Input: part model. Units: mm. Frame: model coordinates. A direction names the side the tool comes from. Round coordinates to 2 decimals unless told otherwise and drop trailing zeros. Write each loop counter-clockwise with the first axis right and the second up, starting at its lowest first coordinate (ties: lowest second). Pieces come first, ordered by that corner, then holes. Notation, with made-up numbers: (72, 28) - (131, 28) arc R17 cw to (131, 60) - close; hole circle Ø9 at (-19, 87.25). An arc over 180 degrees is marked (long way). One line per item, written item: value. Start each with the question number.
```python
from build123d import *

# Parameters (mm, degrees)
SKETCH_1_W      = 82.6
SKETCH_1_H      = 62
EXTRUDE_1_DEPTH = 25
SKETCH_2_W      = 68
SKETCH_2_H      = 12
EXTRUDE_2_DEPTH = 1
FILLET_1_R      = 1
SKETCH_3_R      = 3
EXTRUDE_3_DEPTH = 5.5
SKETCH_4_W      = 10
SKETCH_4_H      = 15
EXTRUDE_4_DEPTH = 11
SKETCH_5_W      = 31
SKETCH_5_H      = 12.5
EXTRUDE_5_DEPTH = 5
EXTRUDE_6_DEPTH = 15
FILLET_2_R      = 1
SKETCH_7_W      = 7
SKETCH_7_H      = 7
EXTRUDE_7_DEPTH = 12.5


with BuildPart() as part:
    # 草图1 → 凸台-拉伸1 (new body)
    with BuildSketch(Plane(origin=(0, 0, 0), x_dir=(1, 0, 0), z_dir=(0, 1, 0))):
        Rectangle(SKETCH_1_W, SKETCH_1_H)
    extrude(amount=EXTRUDE_1_DEPTH)

    # 草图2 → 凸台-拉伸2 (add)
    # profile 1 of 2: a face of its own
    with BuildSketch(Plane.XZ):
        with Locations((0, 37)):
            Rectangle(SKETCH_2_W, SKETCH_2_H)
        with BuildLine():
            Line((-29, 39.5), (-21, 39.5))
            ThreePointArc((-21, 39.5), (-19, 37.5), (-21, 35.5))
            Line((-21, 35.5), (-29, 35.5))
            ThreePointArc((-29, 35.5), (-31, 37.5), (-29, 39.5))
        make_face(mode=Mode.SUBTRACT)
        with BuildLine():
            Line((21, 39.5), (29, 39.5))
            ThreePointArc((29, 39.5), (31, 37.5), (29, 35.5))
            Line((29, 35.5), (21, 35.5))
            ThreePointArc((21, 35.5), (19, 37.5), (21, 39.5))
        make_face(mode=Mode.SUBTRACT)
        with BuildLine():
            Line((-5.5, 39.5), (-2, 39.5))
            ThreePointArc((-2, 39.5), (0, 41.5), (2, 39.5))
            Line((2, 39.5), (5.5, 39.5))
            ThreePointArc((5.5, 39.5), (7.5, 37.5), (5.5, 35.5))
            Line((5.5, 35.5), (2, 35.5))
            ThreePointArc((2, 35.5), (0, 33.5), (-2, 35.5))
            Line((-2, 35.5), (-5.5, 35.5))
            ThreePointArc((-5.5, 35.5), (-7.5, 37.5), (-5.5, 39.5))
        make_face(mode=Mode.SUBTRACT)
    # profile 2 of 2: a face of its own
    with BuildSketch(Plane.XZ):
        with Locations((0, -37)):
            Rectangle(SKETCH_2_W, SKETCH_2_H)
        with BuildLine():
            Line((2, -35.5), (5.5, -35.5))
            ThreePointArc((5.5, -35.5), (7.5, -37.5), (5.5, -39.5))
            Line((5.5, -39.5), (2, -39.5))
            ThreePointArc((2, -39.5), (0, -41.5), (-2, -39.5))
            Line((-2, -39.5), (-5.5, -39.5))
            ThreePointArc((-5.5, -39.5), (-7.5, -37.5), (-5.5, -35.5))
            Line((-5.5, -35.5), (-2, -35.5))
            ThreePointArc((-2, -35.5), (0, -33.5), (2, -35.5))
        make_face(mode=Mode.SUBTRACT)
        with BuildLine():
            Line((21, -39.5), (29, -39.5))
            ThreePointArc((29, -39.5), (31, -37.5), (29, -35.5))
            Line((29, -35.5), (21, -35.5))
            ThreePointArc((21, -35.5), (19, -37.5), (21, -39.5))
        make_face(mode=Mode.SUBTRACT)
        with BuildLine():
            Line((-29, -39.5), (-21, -39.5))
            ThreePointArc((-21, -39.5), (-19, -37.5), (-21, -35.5))
            Line((-21, -35.5), (-29, -35.5))
            ThreePointArc((-29, -35.5), (-31, -37.5), (-29, -39.5))
        make_face(mode=Mode.SUBTRACT)
    extrude(amount=-EXTRUDE_2_DEPTH)

    # 圆角1
    fillet_1_edges = [part.edges().sort_by_distance(p)[0] for p in [
        (0, 1, 31),
        (0, 1, -31),
    ]]
    fillet(fillet_1_edges, radius=FILLET_1_R)

    # 草图3 → 凸台-拉伸3 (add)
    with BuildSketch(Plane(origin=(41.3, 0, 0), x_dir=(0, 0, -1), z_dir=(1, 0, 0))):
        with Locations(Location((-12.5, 12, 0), (0, 0, 180))):
            Circle(SKETCH_3_R)
    extrude(amount=EXTRUDE_3_DEPTH)

    # 草图4 → 凸台-拉伸4 (add)
    with BuildSketch(Plane(origin=(41.3, 0, 0), x_dir=(0, 0, -1), z_dir=(1, 0, 0))):
        with Locations((3, 14)):
            Rectangle(SKETCH_4_W, SKETCH_4_H)
    extrude(amount=EXTRUDE_4_DEPTH)

    # 草图5 → 凸台-拉伸5 (add)
    with BuildSketch(Plane.ZY.offset(41.3)):
        with Locations((8.5, 13.05)):
            Rectangle(SKETCH_5_W, SKETCH_5_H)
    extrude(amount=EXTRUDE_5_DEPTH)

    # 草图6 → 凸台-拉伸6 (add)
    with BuildSketch(Plane.ZY.offset(46.3)):
        Polygon((-1, 18.3), (18, 18.3), (16.5, 7.8), (0.5, 7.8), align=None)
    extrude(amount=EXTRUDE_6_DEPTH)

    # 圆角2
    fillet_2_edges = [part.edges().sort_by_distance(p)[0] for p in [
        (-53.8, 18.3, -1),
        (-53.8, 7.8, 0.5),
        (-53.8, 7.8, 16.5),
        (-53.8, 18.3, 18),
    ]]
    fillet(fillet_2_edges, radius=FILLET_2_R)

    # 草图7 → 凸台-拉伸7 (add)
    with BuildSketch(Plane(origin=(46.8, 0, 0), x_dir=(0, 0, -1), z_dir=(1, 0, 0))):
        with Locations((-12.5, 12)):
            Rectangle(SKETCH_7_W, SKETCH_7_H)
    extrude(amount=EXTRUDE_7_DEPTH)


solid = part.part
```
Q1. Access query for faces 1 (the flat face through (-54, 7.8, 9)), 2 (the cylindrical face through (44, 11.9, 9.5)), 3 (the flat face through (52.3, 14, -3)), 4 (the flat face through (-44, 13, 24)), 5 (the flat face through (-44, 19.3, 8)). Directions: +Z, -Z, +X, -X, +Y, -Y. A direction counts if a zero-diameter tool reaches every point of the face in a straight line with its end or side. Return the directions, or none.
Q2. Cut plane D-D, the plane z = -19. Output: boundary loops of the cut face in (x, y).
Q3. Cut plane B-B, the plane z = -37.5. Output: boundary loops of the cut face in (x, y).
Q4. Contact query for flat-ended pins moving along their axis: pin 1 Ø1 at (x, y) = (24.5, 12) entering from +Z; pin 2 Ø6 at (x, y) = (-2.5, 4.5) entering from +Z; pin 3 Ø7.5 at (x, y) = (54, 11) entering from -Z. Output: stop coordinate, or through.
Q5. Cut plane C-C, the plane y = 12. Output: boundary loops of the cut face in (x, z).
Q6. Material intervals for probe 1 along X at (y, z) = (16.5, 27); probe 2 along Z at (x, y) = (37, 16.25); probe 3 along Y at (x, z) = (-45, 4), sorted ascending. Write a range as from..to.
Q7. Cut plane A-A, the plane x = -26. Output: boundary loops of the cut face in (y, z), and give its area (3 significant figures).
A:
1. face 1: +Z, -Z, -X, -Y
1. face 2: none
1. face 3: -Z, +X, +Y, -Y
1. face 4: +Z, -X, +Y, -Y
1. face 5: +Z, -Z, -X, +Y
2. outline: (-41.3, 0) - (41.3, 0) - (41.3, 25) - (-41.3, 25) - close
3. outline: (-34, 0) - (-31, 0) - (-31, 1) - (-34, 1) - close; (-19, 0) - (-7.5, 0) - (-7.5, 1) - (-19, 1) - close; (7.5, 0) - (19, 0) - (19, 1) - (7.5, 1) - close; (31, 0) - (34, 0) - (34, 1) - (31, 1) - close
4. pin 1: stops at z = 31
4. pin 2: stops at z = 31.13
4. pin 3: stops at z = -8
5. outline: (-61.3, -0.1) - (-46.3, -0.1) - (-46.3, -7) - (-41.3, -7) - (-41.3, -31) - (41.3, -31) - (41.3, -8) - (52.3, -8) - (52.3, 2) - (41.3, 2) - (41.3, 9.5) - (46.8, 9.5) - (46.8, 9) - (59.3, 9) - (59.3, 16) - (46.8, 16) - (46.8, 15.5) - (41.3, 15.5) - (41.3, 31) - (-41.3, 31) - (-41.3, 24) - (-46.3, 24) - (-46.3, 17.1) - (-61.3, 17.1) - close
6. probe 1: x = -41.3..41.3
6. probe 2: z = -31..31
6. probe 3: y = 6.8..19.3
7. outline: (0, -43) - (1, -43) - (1, -39.5) - (0, -39.5) - close; (0, -35.5) - (1, -35.5) - (1, -32) arc R1 cw to (2, -31) - (25, -31) - (25, 31) - (2, 31) arc R1 cw to (1, 32) - (1, 35.5) - (0, 35.5) - close; (0, 39.5) - (1, 39.5) - (1, 43) - (0, 43) - close
7. area: 1,570 mm²
